Read the model definition and answer for the solid it produces. Units are mm, in the model's axes. Face numbers are marked on the shaded views. Round coordinates to 2 decimals unless told otherwise and drop trailing zeros. Order: outer loops, then holes, each group sorted by start corner. A loop starts at its lowest first (then second) coordinate and runs counter-clockwise, first axis right, second up. Notation, with made-up numbers: (63.25, 56.25) -> (115.25, 56.25) arc R12 cw to (115.25, 69.25) -> close; hole circle Ø9 at (76, 8). An arc over 180 degrees is marked (long way). Answer as a JSON object with one key per item and string values. Group by question number.
Item 1: Consider probe 1 along Z at (x, y) = (5, -25.5); probe 2 along X at (y, z) = (18, 33); probe 3 along Y at (x, z) = (40, 8). Determine where each line is inside the solid, lowest interval first. Write a range as from..to.
Item 2: The mould has two halves that part along Z. Classify the marked faces 1, 2 and 3: pulls with the +Z half, pulls with the -Z half, needs draft (parallel to the pull), parting line crosses it, or undercut.
Item 3: Given P1, Ø1, axis at x = 32, y = -5, coming from the -Z side, flat-ended and moving along its own axis, determine where the tip first touches the part or whether it passes through.
Item 4: Section B-B, the plane x = 1.5 is taken. Write down the section's boundary in (y, z), plus the area to 3 significant figures.
Item 5: Section C-C, the plane x = 28.5 is taken. Write down the section's boundary in (y, z).
Item 6: Section A-A, the plane z = 34 is taken. Write down the section's boundary in (x, y), plus the area to 3 significant figures.
Item 7: Section D-D, the plane z = 4.5 is taken. Write down the section's boundary in (x, y), plus the area to 3 significant figures.
from build123d import *

# Parameters (mm, degrees)
F0_W     = 127
F0_H     = 76.2
F1_DEPTH = 45.72
F2_R     = 9.811364
F3_R     = 8.804224
F4_DEPTH = 3.302
F5_W     = 31.836366
F5_H     = 13.6
F6_DEPTH = 50.8


with BuildPart() as f1:
    # F0 (on Top) → F1 (new body)
    with BuildSketch(Plane.XY):
        Rectangle(F0_W, F0_H)
    extrude(amount=F1_DEPTH)

    # F2
    f2_edges = [f1.edges().sort_by_distance(p)[0] for p in [
        (0, -38.1, 45.72),
        (0, 38.1, 45.72),
        (0, -38.1, 0),
        (0, 38.1, 0),
    ]]
    fillet(f2_edges, radius=F2_R)

    # F3 (on face) → F4 (join)
    with BuildSketch(Plane(origin=(0, 0, 0), x_dir=(1, 0, 0), z_dir=(0, 0, -1))):
        with Locations((33.669599, 15.421356)):
            Circle(F3_R)
    extrude(amount=F4_DEPTH)

    # F5 (on face) → F6 (cut)
    with BuildSketch(Plane.YZ.offset(63.5)):
        with Locations((18.707377, 36.119621)):
            Rectangle(F5_W, F5_H)
    extrude(amount=-F6_DEPTH, mode=Mode.SUBTRACT)


solid = f1.part
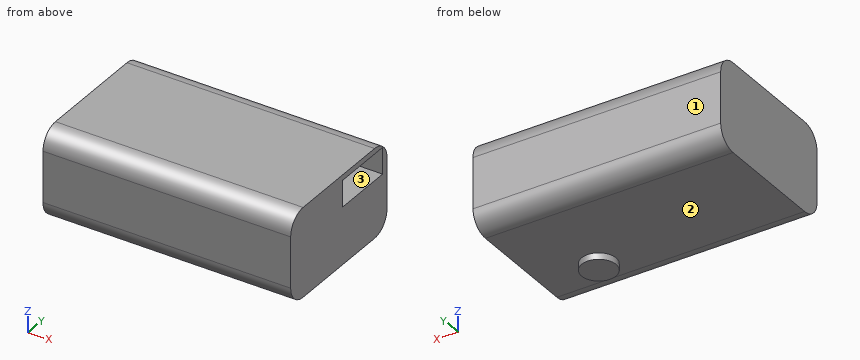
Values found:
{
 "1": {"probe 1": "0..45.72", "probe 2": "-63.5..12.7", "probe 3": "-37.93..37.93"},
 "2": {"face 1": "needs draft", "face 2": "pulls with the -Z half", "face 3": "undercut"},
 "3": {"P1": "z = 0"},
 "4": {"outline": "(-38.1, 9.81) arc R9.81 ccw to (-28.29, 0) -> (28.29, 0) arc R9.81 ccw to (38.1, 9.81) -> (38.1, 35.91) arc R9.81 ccw to (28.29, 45.72) -> (-28.29, 45.72) arc R9.81 ccw to (-38.1, 35.91) -> close", "area": "3,400 mm2"},
 "5": {"outline": "(-38.1, 9.81) arc R9.81 ccw to (-28.29, 0) -> (-22.55, 0) -> (-22.55, -3.3) -> (-8.29, -3.3) -> (-8.29, 0) -> (28.29, 0) arc R9.81 ccw to (38.1, 9.81) -> (38.1, 35.91) arc R9.81 ccw to (28.29, 45.72) -> (-28.29, 45.72) arc R9.81 ccw to (-38.1, 35.91) -> close; hole (2.79, 29.32) -> (34.63, 29.32) -> (34.63, 42.92) -> (2.79, 42.92) -> close"},
 "6": {"outline": "(-63.5, -38.1) -> (63.5, -38.1) -> (63.5, 2.79) -> (12.7, 2.79) -> (12.7, 34.63) -> (63.5, 34.63) -> (63.5, 38.1) -> (-63.5, 38.1) -> close", "area": "8,060 mm2"},
 "7": {"outline": "(-63.5, -36.54) -> (63.5, -36.54) -> (63.5, 36.54) -> (-63.5, 36.54) -> close", "area": "9,280 mm2"}
}
